Input: part model. Units: mm. Frame: model coordinates. Face numbers are marked on the shaded views. A direction names the side the tool comes from. Round coordinates to 2 decimals unless told otherwise and drop trailing zeros. Order: outer loops, then holes, each group sorted by start corner. A loop starts at its lowest first (then second) coordinate and runs counter-clockwise, first axis right, second up.
Item 1: Reachability of the marked faces 1, 2 and 3 from +Z, -Z, +X, -X, +Y, -Y: full face, straight path, thin tool, end or side. Return the list, or none.
Item 2: Cut plane C-C on y = 16.5. Output: boundary loops of the cut face in (x, z), then the cut area to 3 significant figures.
Item 3: Cut plane A-A on z = 0. Output: boundary loops of the cut face in (x, y).
Item 4: Cut plane B-B on x = -9. Output: boundary loops of the cut face in (y, z).
Item 5: Mould query, pull axis X, two halves, no side actions, for the marked faces 4, 5, 6 and 7. Classes: released by +X, released by -X, zero draft, split by the parting line, or undercut.
Item 6: Cut plane D-D on z = 19.5. Output: boundary loops of the cut face in (x, y), then the cut area to 3 significant figures.
Item 7: First-contact query: pin 1 (3 mm diameter, centred on y = 17.5, z = 15.5, fed in from +X); pin 2 (3 mm diameter, centred on x = -9.5, z = 0.5, fed in from -Y); pin 3 (6 mm diameter, centred on x = -4, z = -8.5, fed in from +Y); pin 4 (2 mm diameter, centred on x = 1, y = 53, fed in from -Z). Flat tips, straight axial feed; report the tip coordinate or a pass-through.
Item 8: Line query: L1, parallel to X at y = 1, z = 0; L2, parallel to X at y = 5.5, z = 0; L3, parallel to Z at x = -1.5, y = 47. Output: solid intervals per line, ascending.
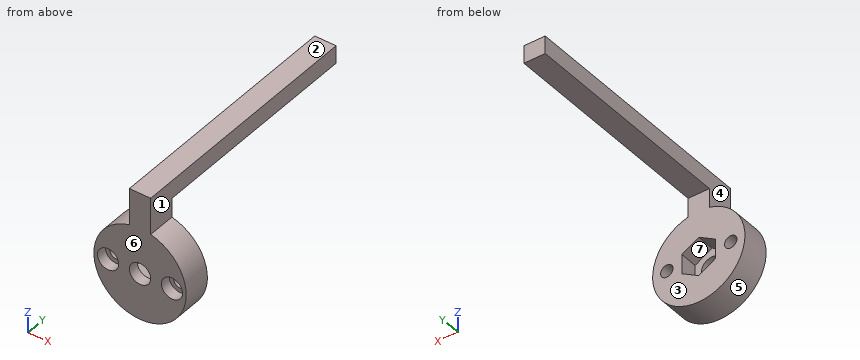
```python
from build123d import *

# Parameters (mm, degrees)
SKETCH1_R           = 13
BOSS_EXTRUDE1_DEPTH = 8
CUT_EXTRUDE1_DEPTH  = 5
SKETCH3_R           = 1.75
CUT_EXTRUDE2_DEPTH  = 21.049937656
SKETCH4_R           = 3
CUT_EXTRUDE3_DEPTH  = 5
SKETCH6_R           = 3
CUT_EXTRUDE4_DEPTH  = 3
SKETCH7_R           = 3
CUT_EXTRUDE5_DEPTH  = 3
SKETCH5_W           = 8
SKETCH5_H           = 6
BOSS_EXTRUDE2_DEPTH = 5
SKETCH8_W           = 6
SKETCH8_H           = 70
BOSS_EXTRUDE3_DEPTH = 5


with BuildPart() as part:
    # Sketch1 → Boss-Extrude1 (new body)
    with BuildSketch(Plane(origin=(0, 0, 0), x_dir=(1, 0, 0), z_dir=(0, 1, 0))):
        with Locations(Location((0, 0, 0), (0, 0, 270))):
            Circle(SKETCH1_R)
    extrude(amount=BOSS_EXTRUDE1_DEPTH)

    # Sketch2 → Cut-Extrude1 (cut)
    with BuildSketch(Plane(origin=(0, 8, 0), x_dir=(1, 0, 0), z_dir=(0, 1, 0))):
        Polygon((0, 5.484827557), (-4.75, 2.742413779), (-4.75, -2.742413779), (0, -5.484827557), (4.75, -2.742413779), (4.75, 2.742413779), align=None)
    extrude(amount=-CUT_EXTRUDE1_DEPTH, mode=Mode.SUBTRACT)

    # Sketch3 → Cut-Extrude2 (cut, through all)
    with BuildSketch(Plane(origin=(0, 8, 0), x_dir=(1, 0, 0), z_dir=(0, 1, 0))):
        with Locations(Location((9, 0, 0), (0, 0, 270))):
            Circle(SKETCH3_R)
    cut_extrude2 = extrude(amount=-CUT_EXTRUDE2_DEPTH, mode=Mode.SUBTRACT)

    # Mirror1: Cut-Extrude2 across plane
    add(cut_extrude2.mirror(Plane(origin=(0, 0, 0), x_dir=(0, 0, 1), z_dir=(1, 0, 0))), mode=Mode.SUBTRACT)

    # Sketch4 → Cut-Extrude3 (cut)
    with BuildSketch(Plane(origin=(0, 3, 0), x_dir=(1, 0, 0), z_dir=(0, 1, 0))):
        with Locations(Location((0, 0, 0), (0, 0, 270))):
            Circle(SKETCH4_R)
    extrude(amount=-CUT_EXTRUDE3_DEPTH, mode=Mode.SUBTRACT)

    # Sketch6 → Cut-Extrude4 (cut)
    with BuildSketch(Plane.XZ):
        with Locations(Location((9, 0, 0), (0, 0, 270))):
            Circle(SKETCH6_R)
    extrude(amount=-CUT_EXTRUDE4_DEPTH, mode=Mode.SUBTRACT)

    # Sketch7 → Cut-Extrude5 (cut)
    with BuildSketch(Plane.XZ):
        with Locations(Location((-9, 0, 0), (0, 0, 270))):
            Circle(SKETCH7_R)
    extrude(amount=-CUT_EXTRUDE5_DEPTH, mode=Mode.SUBTRACT)

    # Sketch5 → Boss-Extrude2 (add, symmetric)
    with BuildSketch(Plane(origin=(0, 0, 13), x_dir=(0, -1, 0), z_dir=(0, 0, 1))):
        with Locations((-4, 0)):
            Rectangle(SKETCH5_W, SKETCH5_H)
    extrude(amount=BOSS_EXTRUDE2_DEPTH, both=True)

    # Sketch8 → Boss-Extrude3 (add)
    with BuildSketch(Plane.XY.offset(18)):
        with Locations((0, 35)):
            Rectangle(SKETCH8_W, SKETCH8_H)
    extrude(amount=BOSS_EXTRUDE3_DEPTH)


solid = part.part
```
From the geometry:
1. face 1: +Z, +X, +Y, -Y
1. face 2: +Z, +X, -X, +Y, -Y
1. face 3: -Z, +X, -X, +Y
2. outline: (-3, 18) - (3, 18) - (3, 23) - (-3, 23) - close
2. area: 30.0 mm2
3. outline: (-13, 0) - (-12, 0) - (-12, 3) - (-10.75, 3) - (-10.75, 8) - (-13, 8) - close; (-7.25, 3) - (-6, 3) - (-6, 0) - (-3, 0) - (-3, 3) - (-4.75, 3) - (-4.75, 8) - (-7.25, 8) - close; (3, 0) - (6, 0) - (6, 3) - (7.25, 3) - (7.25, 8) - (4.75, 8) - (4.75, 3) - (3, 3) - close; (10.75, 3) - (12, 3) - (12, 0) - (13, 0) - (13, 8) - (10.75, 8) - close
4. outline: (0, -9.38) - (8, -9.38) - (8, -1.75) - (3, -1.75) - (3, -3) - (0, -3) - close; (0, 3) - (3, 3) - (3, 1.75) - (8, 1.75) - (8, 9.38) - (0, 9.38) - close
5. face 4: released by -X
5. face 5: split by the parting line
5. face 6: zero draft
5. face 7: undercut
6. outline: (-3, 0) - (3, 0) - (3, 70) - (-3, 70) - close
6. area: 420 mm2
7. pin 1: passes through
7. pin 2: stops at y = 3
7. pin 3: stops at y = 8
7. pin 4: stops at z = 18
8. L1: x = -13 to -12, -6 to -3, 3 to 6, 12 to 13
8. L2: x = -13 to -10.75, -7.25 to -4.75, 4.75 to 7.25, 10.75 to 13
8. L3: z = 18 to 23
